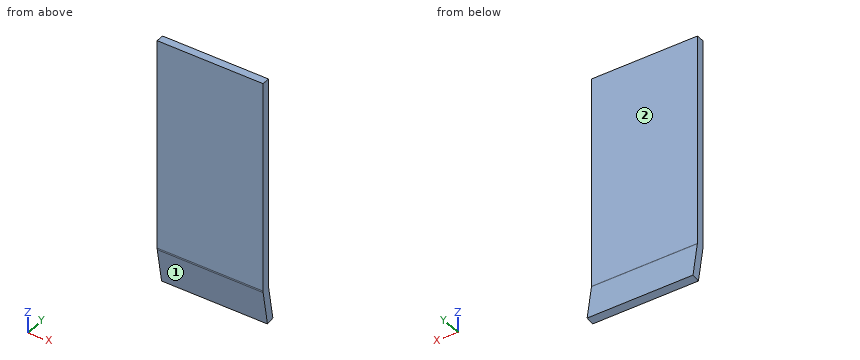
Autodesk Inventor part; units mm, degrees
ref_plane "YZ Plane" through (0, 0, 0) normal (1, 0, 0) x (0, 1, 0)
ref_plane "XZ Plane" through (0, 0, 0) normal (0, 1, 0) x (-1, 0, 0)
ref_plane "XY Plane" through (0, 0, 0) normal (0, 0, 1) x (1, 0, 0)
sketch "Sketch1" plane through (0, 0, 0) normal (0, 1, 0) x (-1, 0, 0)
  line L0 (-10, 20) -> (10, 20)
  line L1 (10, 20) -> (10, -20)
  line L2 (10, -20) -> (-10, -20)
  line L3 (-10, -20) -> (-10, 20)
  line L4 (-10, 20) -> (10, -20) construction
  line L5 (10, 20) -> (-10, -20) construction
  point P0 (0, 0)
  dimension "d0" = 40
  dimension "d1" = 20
extrude "Plate1" add sketch "Sketch1" along normal blind 1.5
sketch "Sketch2" plane through (-10, 1.4772, -19.7395) normal (0, -0.9848078, -0.1736482) x (1, 0, 0)
  line L0 (20, 0) -> (0, 0)
  line L1 (0, 0) -> (0, -7)
  line L2 (0, -7) -> (20, -7)
  line L3 (20, -7) -> (20, 0)
edge flange "Flange1" height 7 angle 10 thickness 1.5 bend radius 0.31 thickness toward (0, -0.9848078, -0.1736482) relief tear relief width 1.5 relief depth 0.75 edges at (0, 1.5, -20) wall of the first edge with corners at (10, 1.4772, -19.7395) (-10, 1.4772, -19.7395) (-10, 2.6927, -26.6332) (10, 2.6927, -26.6332)
bend "Bend1"
corner "Corner1"
equation "\"d2\" = Thickness"
equation "\"d3\" = BendReliefWidth"
equation "\"d4\" = BendReliefDepth"
equation "\"d5\" = MinimumRemnant"
equation "\"d6\" = TransitionRadius"
equation "\"d9\" = BendRadius"
equation "\"d10\" = CornerReliefSize"
equation "\"d11\" = GapSize"
equation "\"d12\" = JacobiRadiusSize"
equation "\"BendReliefWidth\" = Thickness"
equation "\"BendReliefDepth\" = 0.5 * Thickness"
equation "\"CornerReliefSize\" = 4 * Thickness"
equation "\"MinimumRemnant\" = 2 * Thickness"
equation "\"TransitionRadius\" = BendRadius"
equation "\"JacobiRadiusSize\" = BendRadius"
equation "\"GapSize\" = Thickness"
properties part number "axis_23_bottom_frame" material "Aluminum 6061-AHC"
CAD build for the part. Positions are in the model's coordinates, mm. Face numbers are marked on the shaded views. A direction names the side the tool comes from. Round coordinates to 2 decimals unless told otherwise and drop trailing zeros. Loops run counter-clockwise (first coordinate to the right, second up) from the corner with the lowest first, then second, coordinate; pieces in that order, holes last. Notation, with made-up numbers: M 73.5,51 L 88.5,51 A24 ccw 88.5,87 Z; hole C -36.75,66 d5. An arc over 180 degrees is marked long. Return JSON: item names as keys, results as strings. Group by question number.
(1) Tool access for the marked faces 1 and 2: list every direction of +Z, -Z, +X, -X, +Y, -Y with a clear straight run to the whole face (end or side of a thin tool).
(2) Saw through at C-C, the plane y = 0.8. List the corners of the cut face in (x, z), and give its area (3 significant figures).
(3) Drop a flat-ended pin along its axis: P1, Ø6, axis at x = -0.5, z = 7, coming from the +Y side. Give the stop position or say it passes through.
(4) Saw through at A-A, the plane x = -1.5. List the corners of the cut face in (y, z), and give its area (3 significant figures).
(5) Saw through at B-B, the plane z = -16. List the corners of the cut face in (x, y), and give its area (3 significant figures).
(6) Wall check: probe 1 along Y at (x, z) = (4.5, -8.5); probe 2 along Y at (x, z) = (-3.5, -24.5); probe 3 along Z at (x, y) = (-7.5, 1.35). Give the ranges that are in metal, low to high. Write a range as [from, to].
Answer list:
{
 "1": {"face 1": "-Z, +X, -X, -Y", "face 2": "+Z, +X, -X, +Y"},
 "2": {"outline": "M -10,-24.54 L 10,-24.54 L 10,20 L -10,20 Z", "area": "891 mm2"},
 "3": {"P1": "y = 1.5"},
 "4": {"outline": "M 0,-19.84 A1.81 ccw 0.03,-20.16 L 1.22,-26.89 L 2.69,-26.63 L 1.5,-19.9 A0.31 cw 1.5,-19.84 L 1.5,20 L 0,20 Z", "area": "70.3 mm2"},
 "5": {"outline": "M -10,0 L 10,0 L 10,1.5 L -10,1.5 Z", "area": "30.0 mm2"},
 "6": {"probe 1": "[0, 1.5]", "probe 2": "[0.79, 2.32]", "probe 3": "[-26.87, 20]"}
}
